Model file for the job. Use its own axes, mm. Face numbers are marked on the shaded views. A direction names the side the tool comes from. Give positions to 0.01 mm unless a question says otherwise; leave off trailing zeros. Order: outer loops, then holes, each group sorted by start corner. A loop starts at its lowest first (then second) coordinate and runs counter-clockwise, first axis right, second up. Notation, with made-up numbers: (-38.5, -36.75) - (-34.5, -36.75) arc R18 cw to (-34.5, -16.75) - close; hole circle Ø8 at (63.25, 4). An arc over 180 degrees is marked (long way). Return JSON: item names as keys, results as strings. Group by question number.
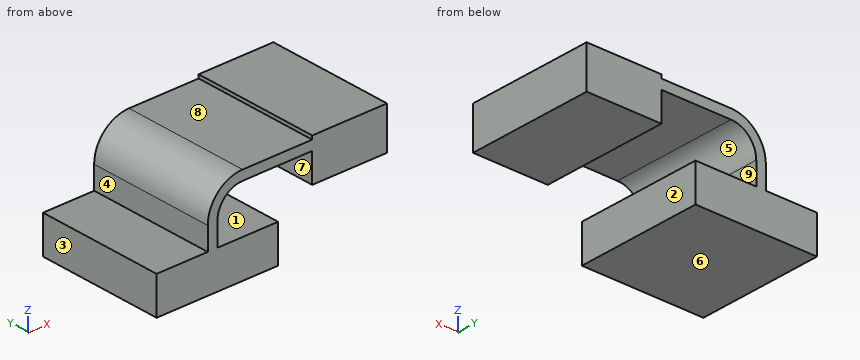
from build123d import *

# Parameters (mm, degrees)
F1_DEPTH = 43.25595


with BuildPart() as f1:
    # F0 (on Front) → F1 (new body, symmetric)
    with BuildSketch(Plane.XZ):
        with BuildLine():
            Line((-6.523012, 28.022824), (-6.523012, 12.7))
            Line((-6.523012, 12.7), (0, 12.7))
            Line((0, 12.7), (0, 28.022824))
            ThreePointArc((0, 28.022824), (5.021654, 40.14617), (17.145, 45.167824))
            Line((17.145, 45.167824), (64.466302, 45.167824))
            Line((64.466302, 45.167824), (64.466302, 51.690836))
            Line((64.466302, 51.690836), (17.145, 51.690836))
            ThreePointArc((17.145, 51.690836), (0.409188, 44.758636), (-6.523012, 28.022824))
        make_face()
        Polygon((-6.523012, 12.7), (-41.275, 12.7), (-41.275, -12.7), (41.275, -12.7), (41.275, 12.7), (0, 12.7), align=None)
        Polygon((64.466302, 54.113042), (64.466302, 51.690836), (64.466302, 45.167824), (64.466302, 25.538042), (115.266302, 25.538042), (115.266302, 54.113042), align=None)
    extrude(amount=F1_DEPTH, both=True)


solid = f1.part
(1) Pull direction Z, two halves, no side cores. Call the marked faces 6, 7, 8 and 9: released by +Z, released by -Z, zero draft, split by the parting line, or undercut.
(2) Slice it at D-D (z = 22.5). Give the cut face in (x, y), and give its area (3 significant figures).
(3) Drill centre lines: L1, parallel to X at y = -38, z = 27.5; L2, parallel to Z at x = 101, y = 3; L3, parallel to X at y = 29, z = 43.5. Where is each one in solid material? Low to high.
(4) Drop flat-ended pins along their axis: pin 1 Ø2 at (x, y) = (63.5, 24) entering from -Z; pin 2 Ø10 at (y, z) = (-18, 21.5) entering from -X; pin 3 Ø4 at (y, z) = (29, 6.5) entering from +X (3 decimals); pin 4 Ø6 at (x, z) = (98, 24.5) entering from +Y. Give the stop position or say it passes through.
(5) 3-axis set-ups, long thin cutter, end or side, ignore diameter. For the marked faces 1, 2, 3, 4 and 5: which of +Z, -Z, +X, -X, +Y, -Y reach the whole face in a straight line?
(6) Slice it at A-A (x = 21). Give the cut face in (y, z).
(7) Slice it at B-B (z = 36). Give the cut face in (x, y).
(8) Slice it at C-C (y = -7). Give the cut face in (x, z) (3 decimals), and give its area (3 significant figures).
Result set:
{
 "1": {"face 6": "released by -Z", "face 7": "zero draft", "face 8": "released by +Z", "face 9": "undercut"},
 "2": {"outline": "(-6.52, -43.26) - (0, -43.26) - (0, 43.26) - (-6.52, 43.26) - close", "area": "564 mm²"},
 "3": {"L1": "x = -6.52 to 0, 64.47 to 115.27", "L2": "z = 25.54 to 54.11", "L3": "x = -0.76 to 9.77, 64.47 to 115.27"},
 "4": {"pin 1": "stops at z = 25.54", "pin 2": "stops at x = -6.52", "pin 3": "stops at x = 41.275", "pin 4": "stops at y = 43.26"},
 "5": {"face 1": "+X, +Y, -Y", "face 2": "-Z, +X, +Y, -Y", "face 3": "+Z, -Z, -X, +Y, -Y", "face 4": "+Z, -X, +Y, -Y", "face 5": "+Y, -Y"},
 "6": {"outline": "(-43.26, -12.7) - (43.26, -12.7) - (43.26, 12.7) - (-43.26, 12.7) - close; (-43.26, 45.17) - (43.26, 45.17) - (43.26, 51.69) - (-43.26, 51.69) - close"},
 "7": {"outline": "(-5.14, -43.26) - (1.97, -43.26) - (1.97, 43.26) - (-5.14, 43.26) - close; (64.47, -43.26) - (115.27, -43.26) - (115.27, 43.26) - (64.47, 43.26) - close"},
 "8": {"outline": "(-41.275, -12.7) - (41.275, -12.7) - (41.275, 12.7) - (0, 12.7) - (0, 28.023) arc R17.145 cw to (17.145, 45.168) - (64.466, 45.168) - (64.466, 25.538) - (115.266, 25.538) - (115.266, 54.113) - (64.466, 54.113) - (64.466, 51.691) - (17.145, 51.691) arc R23.668 ccw to (-6.523, 28.023) - (-6.523, 12.7) - (-41.275, 12.7) - close", "area": "4,170 mm²"}
}
